Here's how the part is built. I have some questions about the finished solid (model axes, mm). Round coordinates to 2 decimals unless told otherwise and drop trailing zeros. Write each loop counter-clockwise with the first axis right and the second up, starting at its lowest first coordinate (ties: lowest second). Pieces come first, ordered by that corner, then holes. Notation, with made-up numbers: (17.25, 60.25) - (72.25, 60.25) arc R36 ccw to (72.25, 97.25) - close; hole circle Ø6 at (74.5, 81). An arc over 180 degrees is marked (long way). Use one line per item in the form item = value. Start each with the question number.
1. If I drill on line 1 along Y through (x, z) = (56, -158.5); line 2 along Z through (x, y) = (59, -46); line 3 along Z through (x, y) = (66, -86.5), over which ranges is the centre line in solid material (lowest first)?
2. I want a section at B-B, the plane z = -158. List the corners of the cut face in (x, y) for me.
3. I want a section at A-A, the plane y = -57. List the corners of the cut face in (x, z) for me, plus the area to 3 significant figures.
4. Will these pins go through, and if not, where does the flat tip stop? pin 1 (8.5 mm diameter, centred on x = 60, z = -154.5, fed in from -Y); pin 2 (4 mm diameter, centred on y = -48.5, z = -106, fed in from +X); pin 3 (4 mm diameter, centred on x = 121.5, y = -62.5, fed in from +Z).
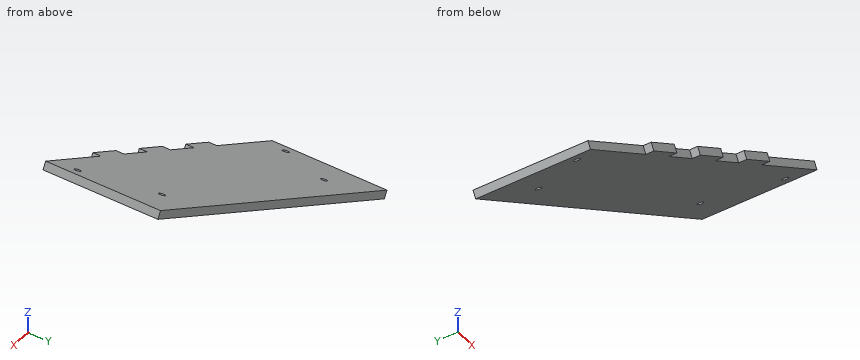
```python
from build123d import *

# Parameters (mm, degrees)
STOCK_FRAME_MASTER_1_START     = 163.456714755
STOCK_FRAME_MASTER_1_OUTLINE_R = 2
STOCK_FRAME_MASTER_1_DEPTH     = 5


# Read off the part's stored shape, not the designer's step: Stock-frame-master-1
with BuildPart() as part:
    # Stock-frame-master-1 outline → Stock-frame-master-1 (new body)
    with BuildSketch(Plane(origin=(0, 0, 0), x_dir=(0.866025403784438, 0, 0.500000000000001), z_dir=(0.500000000000001, 0, -0.866025403784438)).offset(STOCK_FRAME_MASTER_1_START)):
        Polygon((0, 15), (121.884572681, 15), (121.884572681, 89.75), (62.4, 89.75), (62.4, 95), (37.6, 95), (37.6, 89.75), (12.4, 89.75), (12.4, 95), (0, 95), align=None)
        with Locations((87.134572681, 35)):
            Circle(STOCK_FRAME_MASTER_1_OUTLINE_R, mode=Mode.SUBTRACT)
        with Locations((112.134572681, 75)):
            Circle(STOCK_FRAME_MASTER_1_OUTLINE_R, mode=Mode.SUBTRACT)
    extrude(amount=STOCK_FRAME_MASTER_1_DEPTH)

    # Mirror1: part across plane


with BuildPart() as part_1:
    add(part.part)
    add(part.part.mirror(Plane(origin=(81.728357378, -89.75, -141.557667397), x_dir=(-0.5000000000000008, 0, 0.8660254037844382), z_dir=(-0.8660254037844383, 0, -0.5000000000000008))))


solid = part_1.part
```
Model answer:
q1.line_1 = -89.75 to -15
q1.line_2 = -160.45 to -154.68
q1.line_3 = -156.41 to -150.64
q2.outline = (53.25, -89.75) - (63.25, -89.75) - (63.25, -15) - (53.25, -15) - close
q3.outline = (-23.83, -202.5) - (-21.33, -206.83) - (189.78, -84.95) - (187.28, -80.62) - close
q3.area = 1,220 mm2
q4.pin_1 = -89.75
q4.pin_2 = 156.78
q4.pin_3 = -117.44
